from build123d import *

# Parameters (mm, degrees)
F0_W      = 42
F0_H      = 42
F1_DEPTH  = 42
F2_W      = 21
F2_H      = 21
F3_DEPTH  = 42
F4_W      = 21
F4_H      = 21
F5_DEPTH  = 21
F6_W      = 21
F6_H      = 21
F7_DEPTH  = 21
F8_W      = 19
F8_H      = 19
F9_DEPTH  = 41
F10_W     = 19
F10_H     = 19
F11_DEPTH = 41
F12_W     = 19
F12_H     = 19
F13_DEPTH = 41


with BuildPart() as f1:
    # F0 (on Top) → F1 (new body)
    with BuildSketch(Plane.XY):
        Rectangle(F0_W, F0_H)
    extrude(amount=F1_DEPTH)

    # F2 (on face) → F3 (cut, through all)
    with BuildSketch(Plane.XY.offset(42)):
        with Locations((-10.5, 10.5)):
            Rectangle(F2_W, F2_H)
    extrude(amount=-F3_DEPTH, mode=Mode.SUBTRACT)

    # F4 (on face) → F5 (cut, through all)
    with BuildSketch(Plane.XZ.offset(21)):
        with Locations((-10.5, 31.5)):
            Rectangle(F4_W, F4_H)
    extrude(amount=-F5_DEPTH, mode=Mode.SUBTRACT)

    # F6 (on face) → F7 (cut, through all)
    with BuildSketch(Plane.YZ.offset(21)):
        with Locations((10.5, 31.5)):
            Rectangle(F6_W, F6_H)
    extrude(amount=-F7_DEPTH, mode=Mode.SUBTRACT)

    # F8 (on face) → F9 (cut)
    with BuildSketch(Plane.XY.offset(42)):
        with Locations((10.5, -10.5)):
            Rectangle(F8_W, F8_H)
    extrude(amount=-F9_DEPTH, mode=Mode.SUBTRACT)

    # F10 (on face) → F11 (cut)
    with BuildSketch(Plane(origin=(-21, 0, 0), x_dir=(0, -1, 0), z_dir=(-1, 0, 0))):
        with Locations((10.5, 10.5)):
            Rectangle(F10_W, F10_H)
    extrude(amount=-F11_DEPTH, mode=Mode.SUBTRACT)

    # F12 (on face) → F13 (cut)
    with BuildSketch(Plane(origin=(0, 21, 0), x_dir=(-1, 0, 0), z_dir=(0, 1, 0))):
        with Locations((-10.5, 10.5)):
            Rectangle(F12_W, F12_H)
    extrude(amount=-F13_DEPTH, mode=Mode.SUBTRACT)


solid = f1.part
Verification items for the finished model (mm, model axes). A direction names the side the tool comes from. Coordinates: 2 decimals unless noted, no trailing zeros. Write each loop counter-clockwise with the first axis right and the second up, starting at its lowest first coordinate (ties: lowest second). Pieces come first, ordered by that corner, then holes. Notation, with made-up numbers: M -25,-12.5 L 21,-12.5 A17 ccw 21,6.5 Z; hole C -23,83 d1. An arc over 180 degrees is marked long. Use a Markdown table: item, result.
Q1. Draft check along Y on faces 1 (the face through (20, -4, 17)), 2 (the face through (-11, 0, 11)), 3 (the face through (21, -5, 16)). Enter one of: +Y half, -Y half, draft (parallel to the pull), parting line (faces both ways), or undercut.
Reply:
| item | result |
|---|---|
| face 1 | undercut |
| face 2 | +Y half |
| face 3 | draft |
Q2. Go/stop test with flat-tipped pins: P1, Ø3, axis at y = -14, z = 11.5, coming from the -X side; P2, Ø6.5, axis at x = -12.5, z = 6, coming from the +Y side; P3, Ø17, axis at x = 7, y = 12, coming from the +Z side; P4, Ø2, axis at y = 2.5, z = 32, coming from the -X side. Record where each tip stops, or that it passes through.
Reply:
| item | result |
|---|---|
| P1 | stops at x = 20 |
| P2 | stops at y = 0 |
| P3 | stops at z = 21 |
| P4 | passes through |
Q3. Sectioned sample at A-A, the plane z = 4. Record the boundary of the cut face in (x, y), plus the area to 3 significant figures.
Reply:
| item | result |
|---|---|
| outline | M -21,-21 L 21,-21 L 21,21 L 20,21 L 20,-20 L -21,-20 Z; M -21,-1 L 1,-1 L 1,21 L 0,21 L 0,0 L -21,0 Z |
| area | 126 mm² |
Q4. Sectioned sample at B-B, the plane y = -9.5. Record the boundary of the cut face in (x, z).
Reply:
| item | result |
|---|---|
| outline | M -21,0 L 21,0 L 21,42 L 20,42 L 20,1 L -21,1 Z; M -21,20 L 1,20 L 1,42 L 0,42 L 0,21 L -21,21 Z |
Q5. Sectioned sample at C-C, the plane z = 33.5. Record the boundary of the cut face in (x, y).
Reply:
| item | result |
|---|---|
| outline | M 0,-21 L 21,-21 L 21,0 L 0,0 Z; hole M 1,-20 L 20,-20 L 20,-1 L 1,-1 Z |
Q6. Set-up check for faces 4 (the face through (4, -4, 1)), 5 (the face through (10, -1, 31)), 6 (the face through (-10, -10, 20)): record each of +Z, -Z, +X, -X, +Y, -Y from which the full face is reachable in a straight line by a thin tool's end or side.
Reply:
| item | result |
|---|---|
| face 4 | none |
| face 5 | +Z |
| face 6 | -X |
Q7. Sectioned sample at D-D, the plane y = 18. Record the boundary of the cut face in (x, z).
Reply:
| item | result |
|---|---|
| outline | M 0,0 L 21,0 L 21,21 L 0,21 Z; hole M 1,1 L 20,1 L 20,20 L 1,20 Z |
Q8. Thickness scan on line 1 (X direction, y = 5, z = 5.5); line 2 (Y direction, x = -16.5, z = 4). Record the ranges inside material, lowest first.
Reply:
| item | result |
|---|---|
| line 1 | x = 0 to 1, 20 to 21 |
| line 2 | y = -21 to -20, -1 to 0 |
